from build123d import *

# Parameters (mm, degrees)
SKETCH_1_W          = 150
SKETCH_1_H          = 100
EXTRUDE_1_DEPTH     = 65
SKETCH_4_W          = 140
SKETCH_4_H          = 90
CUT_EXTRUDE_1_DEPTH = 55
SKETCH_5_R          = 38
EXTRUDE_2_DEPTH     = 30


with BuildPart() as part:
    # 草图1 → 凸台-拉伸1 (new body)
    with BuildSketch(Plane.XY):
        Rectangle(SKETCH_1_W, SKETCH_1_H)
    extrude(amount=EXTRUDE_1_DEPTH)

    # 草图4 → 切除-拉伸1 (cut)
    with BuildSketch(Plane.XY.offset(60)):
        Rectangle(SKETCH_4_W, SKETCH_4_H)
    extrude(amount=-CUT_EXTRUDE_1_DEPTH, mode=Mode.SUBTRACT)

    # 草图5 → 凸台-拉伸2 (add)
    with BuildSketch(Plane(origin=(0, 0, 0), x_dir=(-1, 0, 0), z_dir=(0, 0, -1))):
        with Locations(Location((0, 0, 0), (0, 0, 180))):
            Circle(SKETCH_5_R)
    extrude(amount=EXTRUDE_2_DEPTH)


solid = part.part
The listing builds one solid part. Answer for the finished solid, in the listing's coordinates (mm). A direction names the side the tool comes from. Give positions to 0.01 mm unless a question says otherwise; leave off trailing zeros. Order: outer loops, then holes, each group sorted by start corner. A loop starts at its lowest first (then second) coordinate and runs counter-clockwise, first axis right, second up. Notation, with made-up numbers: (24, 11) - (70, 11) arc R30 cw to (70, 42) - close; hole circle Ø9 at (37, 35.5). An arc over 180 degrees is marked (long way). Use one line per item in the form item = value.
1) For faces 1 (the flat face through (-1, -50, 32)), 2 (the flat face through (-1, -45, 33)), 3 (the flat face through (-18, 34, 0)), determine the directions among +Z, -Z, +X, -X, +Y, -Y from which every point of the face is accessible in a straight line to the end or side of a thin tool.
Verdict:
face_1 = +Z, -Z, +X, -X, -Y
face_2 = none
face_3 = -Z
2) Find section C-C on y = 0. Determine the outline of the cut face in (x, z).
Verdict:
outline = (-75, 0) - (-38, 0) - (-38, -30) - (38, -30) - (38, 0) - (75, 0) - (75, 65) - (-75, 65) - close; hole (-70, 5) - (70, 5) - (70, 60) - (-70, 60) - close
3) Find section A-A on x = 0. Determine the outline of the cut face in (y, z), and give its area (3 significant figures).
Verdict:
outline = (-50, 0) - (-38, 0) - (-38, -30) - (38, -30) - (38, 0) - (50, 0) - (50, 65) - (-50, 65) - close; hole (-45, 5) - (45, 5) - (45, 60) - (-45, 60) - close
area = 3,830 mm^2
4) Find section D-D on x = -40.5. Determine the outline of the cut face in (y, z), and give its area (3 significant figures).
Verdict:
outline = (-50, 0) - (50, 0) - (50, 65) - (-50, 65) - close; hole (-45, 5) - (45, 5) - (45, 60) - (-45, 60) - close
area = 1,550 mm^2
5) This flat-tipped pin is pushed along its axis until it touches: pin 1 (2 mm diameter, centred on y = 20, z = -9, fed in from +X). Where does it stop, or does it pass through?
Verdict:
pin_1 = 32.91
6) Consider probe 1 along Z at (x, y) = (-69, -10); probe 2 along Y at (x, z) = (4.5, 54); probe 3 along Z at (x, y) = (-37, 8). Determine where each line is inside the solid, lowest interval first. Write a range as [from, to].
Verdict:
probe_1 = [0, 5], [60, 65]
probe_2 = [-50, -45], [45, 50]
probe_3 = [-30, 5], [60, 65]
7) Find section B-B on z = 32.5. Determine the outline of the cut face in (x, y).
Verdict:
outline = (-75, -50) - (75, -50) - (75, 50) - (-75, 50) - close; hole (-70, -45) - (70, -45) - (70, 45) - (-70, 45) - close
8) The mould has two halves that part along X. Classify faces 4 (the flat face through (-1, 1, 60)), 5 (the flat face through (75, -1, 32)), 6 (the flat face through (-1, 50, 32)): released by +X, released by -X, zero draft, split by the parting line, or undercut.
Verdict:
face_4 = undercut
face_5 = released by +X
face_6 = zero draft
